Here's how the part is built. I have some questions about the finished solid (model axes, mm). A direction names the side the tool comes from. Coordinates: 2 decimals unless noted, no trailing zeros. Write each loop counter-clockwise with the first axis right and the second up, starting at its lowest first coordinate (ties: lowest second). Pieces come first, ordered by that corner, then holes.
Item 1: I want a section at C-C (z = -13.5). Please give me the cut outline in (x, y).
Item 2: Please list where these lines run through material, in increasing order: line 1 (X direction, y = -4.25, z = -21.5); line 2 (Y direction, x = 0, z = 2); line 3 (Z direction, x = 21.5, y = 9).
Item 3: I'm going to push flat-ended pins straight in: P1, Ø6, axis at x = 4, y = -1.5, coming from the -Z side; P2, Ø6, axis at x = -18, z = -20.5, coming from the +Y side; P3, Ø4, axis at y = 10, z = -14, coming from the -X side; P4, Ø4.5, axis at x = 0, y = -11, coming from the +Z side. Where does each tip first touch, or does it pass through?
Item 4: For faces 5 (the face through (10, 0, -15)), 6 (the face through (-19, -8, 2)), 7 (the face through (19, -8, 2)), 8 (the face through (17, 2, -7)), which set-ups out of +Z, -Z, +X, -X, +Y, -Y let a thin tool reach every point of the face, with its end or its side?
Item 5: If we mould it in two halves opening along X, with no side actions, what happens to faces 1 (the face through (14, -8, -14)), 2 (the face through (-10, 0, -15)), 3 (the face through (-19, 0, -14)), 4 (the face through (-17, 2, -7))? For each: pulls with the +X half, pulls with the -X half, needs draft (parallel to the pull), parting line crosses it, or undercut.
Item 6: I want a section at B-B (y = -11). Please give me the cut outline in (x, z), and give its area (3 significant figures).
Item 7: I want a section at D-D (x = 15). Please give me the cut outline in (y, z), and give its area (3 significant figures).
Item 8: I want a section at A-A (x = 0). Please give me the cut outline in (y, z), and give its area (3 significant figures).
from build123d import *

# Parameters (mm, degrees)
BOSS_EXTRUDE1_DEPTH = 15
BOSS_EXTRUDE2_DEPTH = 2
SKETCH3_R           = 2
CUT_EXTRUDE1_DEPTH  = 42.243181255


with BuildPart() as part:
    # Sketch1 → Boss-Extrude1 (new, symmetric)
    with BuildSketch(Plane(origin=(0, 0, 0), x_dir=(1, 0, 0), z_dir=(0, 1, 0))):
        Polygon((10, 0), (-10, 0), (-10, 30), (-14, 30), (-14, -2), (-24, -2), (-24, -6), (24, -6), (24, -2), (14, -2), (14, 30), (10, 30), align=None)
    extrude(amount=BOSS_EXTRUDE1_DEPTH, both=True)

    # Sketch2 → Boss-Extrude2 (add, symmetric)
    with BuildSketch(Plane(origin=(0, 0, 0), x_dir=(1, 0, 0), z_dir=(0, 1, 0))):
        Polygon((14, 30), (14, -2), (24, -2), align=None)
    boss_extrude2 = extrude(amount=BOSS_EXTRUDE2_DEPTH, both=True)

    # Mirror1: Boss-Extrude2 across plane
    add(boss_extrude2.mirror(Plane(origin=(0, 0, 0), x_dir=(0, 0, 1), z_dir=(1, 0, 0))))

    # Sketch3 → Cut-Extrude1 (cut, through all)
    with BuildSketch(Plane(origin=(0, 0, 0), x_dir=(-1, 0, 0), z_dir=(0, 0, -1))):
        with Locations((0, -11)):
            Circle(SKETCH3_R)
    extrude(amount=-CUT_EXTRUDE1_DEPTH, mode=Mode.SUBTRACT)


solid = part.part
Answer:
1. outline: (-19.16, -2) - (-14, -2) - (-14, -15) - (-10, -15) - (-10, 15) - (-14, 15) - (-14, 2) - (-19.16, 2) - close; (10, -15) - (14, -15) - (14, -2) - (19.16, -2) - (19.16, 2) - (14, 2) - (14, 15) - (10, 15) - close
2. line 1: x = -14 to -10, 10 to 14
2. line 2: y = -15 to -13, -9 to 15
2. line 3: z = 2 to 6
3. P1: stops at z = 0
3. P2: stops at y = 2
3. P3: stops at x = -14
3. P4: stops at z = 6
4. face 5: -Z, +Y, -Y
4. face 6: -Z, -X, -Y
4. face 7: -Z, +X, -Y
4. face 8: -Z, +X, +Y
5. face 1: pulls with the +X half
5. face 2: undercut
5. face 3: pulls with the -X half
5. face 4: needs draft
6. outline: (-24, 2) - (-14, 2) - (-14, -30) - (-10, -30) - (-10, 0) - (-2, 0) - (-2, 6) - (-24, 6) - close; (2, 0) - (10, 0) - (10, -30) - (14, -30) - (14, 2) - (24, 2) - (24, 6) - (2, 6) - close
6. area: 464 mm2
7. outline: (-15, 2) - (-2, 2) - (-2, -26.8) - (2, -26.8) - (2, 2) - (15, 2) - (15, 6) - (-15, 6) - close
7. area: 235 mm2
8. outline: (-15, 0) - (-13, 0) - (-13, 6) - (-15, 6) - close; (-9, 0) - (15, 0) - (15, 6) - (-9, 6) - close
8. area: 156 mm2
